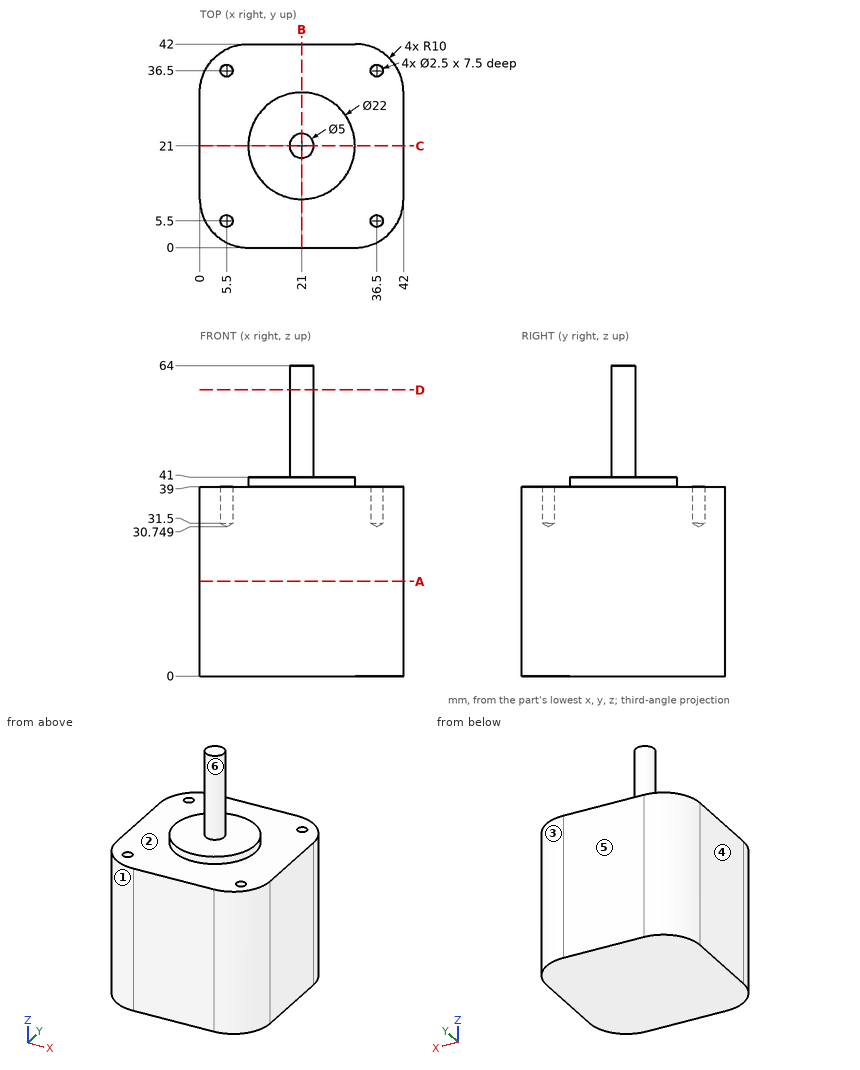
For this review, use the dimensioned drawing (mm, ordinates from the lowest corner) and the shaded views. A direction names the side the tool comes from. Round coordinates to 2 decimals unless told otherwise and drop trailing zeros. Write each loop counter-clockwise with the first axis right and the second up, starting at its lowest first coordinate (ties: lowest second). Pieces come first, ordered by that corner, then holes. Notation, with made-up numbers: (20.25, -31.75) - (33.25, -31.75) arc R23 ccw to (33.25, 6.25) - close; hole circle Ø7 at (-0.75, 23). An arc over 180 degrees is marked (long way). Use a Markdown table: item, result.
Q1. We need section A-A (z = 19.5). Give the boundary of the cut face in (x, y), plus the area to 3 significant figures.
Derived:
| item | result |
|---|---|
| outline | (0, 10) arc R10 ccw to (10, 0) - (32, 0) arc R10 ccw to (42, 10) - (42, 32) arc R10 ccw to (32, 42) - (10, 42) arc R10 ccw to (0, 32) - close |
| area | 1,680 mm2 |
Q2. Wall thickness on line 1 along Y through (x, z) = (5.5, 35); line 2 along Y through (x, z) = (36, 36) (1 decimal): over which ranges is each line inside the solid? List them lowest first.
Derived:
| item | result |
|---|---|
| line 1 | y = 1.07 to 4.25, 6.75 to 35.25, 37.75 to 40.93 |
| line 2 | y = 0.8 to 4.4, 6.6 to 35.4, 37.6 to 41.2 |
Q3. Clearance check with flat-ended pins moving along their axes: pin 1 (8 mm diameter, centred on y = 37.5, z = 17, fed in from -X); pin 2 (1 mm diameter, centred on x = 21.5, y = 26.5, fed in from +Z); pin 3 (2 mm diameter, centred on x = 5.5, y = 5.5, fed in from +Z). State where each tip first meets the part, or that it passes through.
Derived:
| item | result |
|---|---|
| pin 1 | stops at x = 0.11 |
| pin 2 | stops at z = 41 |
| pin 3 | stops at z = 31.35 |
Q4. Machinability: for the marked faces 1 and 2, which of the approach directions +Z, -Z, +X, -X, +Y, -Y give a long, thin tool a straight path to every point of the face, cutting with its end or side? Answer none if there is none.
Derived:
| item | result |
|---|---|
| face 1 | +Z, -Z, -X, -Y |
| face 2 | +Z |
Q5. We need section B-B (x = 21). Give the boundary of the cut face in (y, z).
Derived:
| item | result |
|---|---|
| outline | (0, 0) - (42, 0) - (42, 39) - (32, 39) - (32, 41) - (23.5, 41) - (23.5, 64) - (18.5, 64) - (18.5, 41) - (10, 41) - (10, 39) - (0, 39) - close |
Q6. The part is to be moulded in two halves that separate along X. For the marked faces 3, 4, 5 and 6, say which applies: pulls with the +X half, pulls with the -X half, needs draft (parallel to the pull), parting line crosses it, or undercut.
Derived:
| item | result |
|---|---|
| face 3 | pulls with the +X half |
| face 4 | pulls with the -X half |
| face 5 | needs draft |
| face 6 | parting line crosses it |
Q7. We need section D-D (z = 59). Give the boundary of the cut face in (x, y), plus the area to 3 significant figures.
Derived:
| item | result |
|---|---|
| outline | circle Ø5 at (21, 21) |
| area | 19.6 mm2 |
